Build history of the part. All positions in model axes, mm. Face numbers are marked on the shaded views. A direction names the side the tool comes from. Give positions to 0.01 mm unless a question says otherwise; leave off trailing zeros. Write each loop counter-clockwise with the first axis right and the second up, starting at its lowest first coordinate (ties: lowest second). Pieces come first, ordered by that corner, then holes.
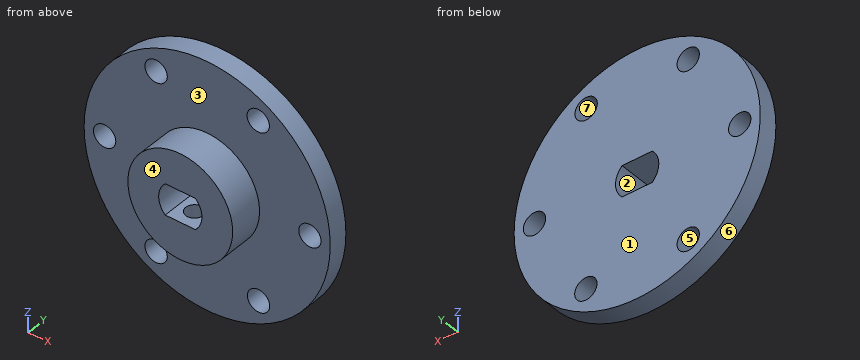
from build123d import *

# Parameters (mm, degrees)
F0_R     = 12.1666
F1_DEPTH = 12.446
F0_R_2   = 28.575
F0_R_3   = 2.5908
F2_DEPTH = 4.572
F4_D     = 4.0386
F4_DEPTH = 28.576


with BuildPart() as f1:
    # F0 (on Front) → F1 (new body)
    with BuildSketch(Plane.XZ):
        Circle(F0_R)
        with BuildLine():
            ThreePointArc((-3.5111765908, -3.5917490267), (-5.02285, 0), (-3.5111765908, 3.5917490267))
            Line((-3.5111765908, 3.5917490267), (3.5111765908, 3.5917490267))
            ThreePointArc((3.5111765908, 3.5917490267), (5.02285, 0), (3.5111765908, -3.5917490267))
            Line((3.5111765908, -3.5917490267), (-3.5111765908, -3.5917490267))
        make_face(mode=Mode.SUBTRACT)
    extrude(amount=F1_DEPTH)

    # F0 (on Front) → F2 (join)
    with BuildSketch(Plane.XZ):
        Circle(F0_R_2)
        with Locations((-11.85156133, -20.6537079066)):
            Circle(F0_R_3, mode=Mode.SUBTRACT)
        with Locations((11.9244238196, -20.6537079066)):
            Circle(F0_R_3, mode=Mode.SUBTRACT)
        with Locations((-23.8124163945, 0.063100767)):
            Circle(F0_R_3, mode=Mode.SUBTRACT)
        with Locations((-11.85156133, 20.6537079066)):
            Circle(F0_R_3, mode=Mode.SUBTRACT)
        Circle(F0_R, mode=Mode.SUBTRACT)
        with Locations((23.8488476393, 0)):
            Circle(F0_R_3, mode=Mode.SUBTRACT)
        with Locations((11.85156133, 20.6537079066)):
            Circle(F0_R_3, mode=Mode.SUBTRACT)
    extrude(amount=F2_DEPTH)

    # F4 (through all, one way)
    with BuildSketch(Plane.XY):
        with Locations((0, -8.3013873111)):
            Circle(F4_D / 2)
    extrude(amount=-F4_DEPTH, mode=Mode.SUBTRACT)


solid = f1.part
(1) Drop flat-ended pins along their axis: pin 1 (3 mm diameter, centred on x = 2.5, z = 2, fed in from +Y); pin 2 (10 mm diameter, centred on x = -20, z = -8.5, fed in from -Y); pin 3 (2.5 mm diameter, centred on x = 0, y = -8.3, fed in from -Z); pin 4 (3.5 mm diameter, centred on x = 0, y = -5.5, fed in from +Z) (3 decimals). Give the stop position or say it passes through.
(2) Saw through at B-B, the plane z = -22.5. List the corners of the cut face in (x, y).
(3) 3-axis set-ups, long thin cutter, end or side, ignore diameter. For the marked faces 1, 2 and 3: which of +Z, -Z, +X, -X, +Y, -Y reach the whole face in a straight line?
(4) Probe line 1 (Z direction, x = 10.5, y = -1); line 2 (Y direction, x = -10, z = -14.5); line 3 (X direction, y = -8.25, z = -9). List the from-to ranges inside material, lowest first.
(5) Saw through at C-C, the plane z = -11. List the corners of the cut face in (x, y).
(6) Saw through at D-D, the plane z = 1. List the corners of the cut face in (x, y).
(7) Mould opens along Z. For the marked faces 4, 5, 6 and 7 say: +Z half, -Z half, draft (parallel to the pull), parting line (faces both ways), or undercut.
(8) Saw through at A-A, the plane x = 0. List the corners of the cut face in (y, z) (3 decimals), plus the area to 3 significant figures.
Computed values:
1. pin 1: passes through
1. pin 2: stops at y = -4.57
1. pin 3: stops at z = 3.59
1. pin 4: stops at z = 28.575
2. outline: (-17.61, -4.57) - (-13.67, -4.57) - (-13.67, 0) - (-17.61, 0) - close; (-10.03, -4.57) - (10.11, -4.57) - (10.11, 0) - (-10.03, 0) - close; (13.74, -4.57) - (17.61, -4.57) - (17.61, 0) - (13.74, 0) - close
3. face 1: +Z, -Z, +X, -X, +Y
3. face 2: +Y, -Y
3. face 3: -Y
4. line 1: z = -26.58 to -22.82, -18.49 to 18.44, 22.86 to 26.58
4. line 2: y = -4.57 to 0
4. line 3: x = -8.19 to -2.02, 2.02 to 8.19
5. outline: (-26.37, -4.57) - (-5.2, -4.57) - (-5.2, -12.45) - (5.2, -12.45) - (5.2, -4.57) - (26.37, -4.57) - (26.37, 0) - (-26.37, 0) - close; hole circle Ø4.04 at (0, -8.3)
6. outline: (-28.56, -4.57) - (-26.23, -4.57) - (-26.23, 0) - (-28.56, 0) - close; (-21.4, -4.57) - (-12.13, -4.57) - (-12.13, -12.45) - (-4.92, -12.45) - (-4.92, 0) - (-21.4, 0) - close; (4.92, -12.45) - (12.13, -12.45) - (12.13, -4.57) - (21.46, -4.57) - (21.46, 0) - (4.92, 0) - close; (26.24, -4.57) - (28.56, -4.57) - (28.56, 0) - (26.24, 0) - close
7. face 4: draft
7. face 5: undercut
7. face 6: parting line
7. face 7: undercut
8. outline: (-12.446, -12.167) - (-10.321, -12.167) - (-10.321, -3.592) - (-12.446, -3.592) - close; (-12.446, 3.592) - (0, 3.592) - (0, 28.575) - (-4.572, 28.575) - (-4.572, 12.167) - (-12.446, 12.167) - close; (-6.282, -12.167) - (-4.572, -12.167) - (-4.572, -28.575) - (0, -28.575) - (0, -3.592) - (-6.282, -3.592) - close
8. area: 329 mm2
